```python
from build123d import *

# Parameters (mm, degrees)
SKETCH001_W     = 97.5
SKETCH001_H     = 91
PAD_DEPTH       = 7
SKETCH_W        = 93.5
SKETCH_H        = 87
POCKET_DEPTH    = 5
SKETCH002_W     = 5
SKETCH002_H     = 5
SKETCH002_R     = 1.6
PAD001_DEPTH    = 5
POCKET001_DEPTH = 1.8
SKETCH003_W     = 10
SKETCH003_H     = 26.5
POCKET002_DEPTH = 5
SKETCH004_W     = 21
SKETCH004_H     = 10
POCKET003_DEPTH = 7.001


with BuildPart() as part:
    # Sketch001 → Pad (new body)
    with BuildSketch(Plane.XY):
        with Locations((0, -43.5)):
            Rectangle(SKETCH001_W, SKETCH001_H)
    extrude(amount=-PAD_DEPTH)

    # Sketch → Pocket (cut)
    with BuildSketch(Plane.XY):
        with Locations((0, -43.5)):
            Rectangle(SKETCH_W, SKETCH_H)
    extrude(amount=-POCKET_DEPTH, mode=Mode.SUBTRACT)

    # Sketch002 → Pad001 (join)
    with BuildSketch(Plane.XY):
        with Locations((-44.25, -2.5)):
            Rectangle(SKETCH002_W, SKETCH002_H)
        with Locations((-44.25, -2.5)):
            Circle(SKETCH002_R, mode=Mode.SUBTRACT)
        with Locations((-44.25, -67.5)):
            Rectangle(SKETCH002_W, SKETCH002_H)
        with Locations((-44.25, -67.5)):
            Circle(SKETCH002_R, mode=Mode.SUBTRACT)
        with Locations((44.25, -67.5)):
            Rectangle(SKETCH002_W, SKETCH002_H)
        with Locations((44.25, -67.5)):
            Circle(SKETCH002_R, mode=Mode.SUBTRACT)
        with Locations((44.25, -2.5)):
            Rectangle(SKETCH002_W, SKETCH002_H)
        with Locations((44.25, -2.5)):
            Circle(SKETCH002_R, mode=Mode.SUBTRACT)
    extrude(amount=-PAD001_DEPTH)

    # Sketch → Pocket001 (cut)
    with BuildSketch(Plane.XY):
        with Locations((0, -43.5)):
            Rectangle(SKETCH_W, SKETCH_H)
    extrude(amount=-POCKET001_DEPTH, mode=Mode.SUBTRACT)

    # Sketch003 → Pocket002 (cut)
    with BuildSketch(Plane.XY):
        with Locations((-51.75, -35.25)):
            Rectangle(SKETCH003_W, SKETCH003_H)
    extrude(amount=-POCKET002_DEPTH, mode=Mode.SUBTRACT)

    # Sketch004 → Pocket003 (cut, through all)
    with BuildSketch(Plane.XY):
        with Locations((-15.5, -11.5)):
            Rectangle(SKETCH004_W, SKETCH004_H)
        with Locations((15.5, -11.5)):
            Rectangle(SKETCH004_W, SKETCH004_H)
    extrude(amount=-POCKET003_DEPTH, mode=Mode.SUBTRACT)


solid = part.part
```
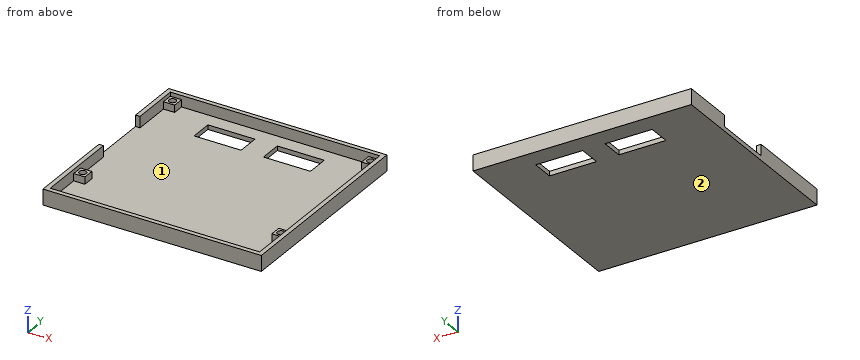
CAD build for the part. Positions are in the model's coordinates, mm. Face numbers are marked on the shaded views. Coordinates: 2 decimals unless noted, no trailing zeros. Write each loop counter-clockwise with the first axis right and the second up, starting at its lowest first coordinate (ties: lowest second). Pieces come first, ordered by that corner, then holes. Notation, with made-up numbers: (-19, 69.5) -> (-13, 69.5) arc R33 ccw to (-13, 97.5) -> close; hole circle Ø10 at (-21.5, 21.25). An arc over 180 degrees is marked (long way). Return JSON: item names as keys, results as strings. Group by question number.
Q1. Cut at B-B, the plane y = -56. Give the cut face in (x, z), then the cut area to 3 significant figures.
Q2. Cut at D-D, the plane z = -3.75. Give the cut face in (x, y), then the cut area to 3 significant figures.
Q3. Cut at A-A, the plane x = 15. Give the cut face in (y, z), then the cut area to 3 significant figures.
Q4. Pull direction X, two halves, no side cores. Call the marked faces 1 and 2: released by +X, released by -X, zero draft, split by the parting line, or undercut.
Q5. Flat gauge pins, fed straight in: pin 1 (1 mm diameter, centred on x = -34.5, y = -80, fed in from +Z); pin 2 (1.5 mm diameter, centred on x = -45, y = -3, fed in from +Z). Where does each tip first touch, or does it go through?
Q6. Drill centre lines: line 1 (Y direction, x = -44.25, z = -3); line 2 (X direction, y = -2, z = -4); line 3 (Y direction, x = -14, z = -4). Where is each one in solid material? Low to high.
Q7. Cut at C-C, the plane x = 29.5. Give the cut face in (y, z).
Returned:
{
 "1": {"outline": "(-48.75, -7) -> (48.75, -7) -> (48.75, 0) -> (46.75, 0) -> (46.75, -5) -> (-46.75, -5) -> (-46.75, 0) -> (-48.75, 0) -> close", "area": "215 mm2"},
 "2": {"outline": "(-48.75, -89) -> (48.75, -89) -> (48.75, 2) -> (-48.75, 2) -> (-48.75, -22) -> (-46.75, -22) -> (-46.75, -5) -> (-41.75, -5) -> (-41.75, 0) -> (41.75, 0) -> (41.75, -5) -> (46.75, -5) -> (46.75, -65) -> (41.75, -65) -> (41.75, -70) -> (46.75, -70) -> (46.75, -87) -> (-46.75, -87) -> (-46.75, -70) -> (-41.75, -70) -> (-41.75, -65) -> (-46.75, -65) -> (-46.75, -48.5) -> (-48.75, -48.5) -> close; hole circle Ø3.2 at (-44.25, -67.5); hole circle Ø3.2 at (-44.25, -2.5); hole circle Ø3.2 at (44.25, -67.5); hole circle Ø3.2 at (44.25, -2.5)", "area": "753 mm2"},
 "3": {"outline": "(-89, -7) -> (-16.5, -7) -> (-16.5, -5) -> (-87, -5) -> (-87, 0) -> (-89, 0) -> close; (-6.5, -7) -> (2, -7) -> (2, 0) -> (0, 0) -> (0, -5) -> (-6.5, -5) -> close", "area": "182 mm2"},
 "4": {"face 1": "undercut", "face 2": "zero draft"},
 "5": {"pin 1": "stops at z = -5", "pin 2": "stops at z = -1.8"},
 "6": {"line 1": "y = -89 to -87, -70 to -69.1, -65.9 to -65, -5 to -4.1, -0.9 to 2", "line 2": "x = -48.75 to -45.77, -42.73 to -41.75, 41.75 to 42.73, 45.77 to 48.75", "line 3": "y = -89 to -87, 0 to 2"},
 "7": {"outline": "(-89, -7) -> (2, -7) -> (2, 0) -> (0, 0) -> (0, -5) -> (-87, -5) -> (-87, 0) -> (-89, 0) -> close"}
}
